```python
from build123d import *

# Parameters (mm, degrees)
AXIAL_PROFILE_MM_W     = 4
AXIAL_PROFILE_MM_H     = 19
AXIAL_HOLES_DEPTH      = 151.487507787
AXIAL_HOLES_DEPTH_BACK = 151.487507787
SKETCH2_R              = 1.25
SKETCH2_R_2            = 1.65


with BuildPart() as part:
    # Axial profile (mm) → Full revolution (revolve)
    with BuildSketch(Plane.XY, mode=Mode.PRIVATE) as full_revolution_sk:
        with Locations((133.7, 36.5)):
            Rectangle(AXIAL_PROFILE_MM_W, AXIAL_PROFILE_MM_H)
    revolve(full_revolution_sk.sketch.rotate(Axis((-110, 0, 0), (1, 0, 0)), 90), axis=Axis((-110, 0, 0), (1, 0, 0)))

    # Sketch2 → Axial holes (cut, two sides: drawn at the far end of the back side and taken through both)
    with BuildSketch(Plane(origin=(0, 0, 0), x_dir=(0, 0, -1), z_dir=(1, 0, 0)).offset(-AXIAL_HOLES_DEPTH_BACK)):
        with Locations((0, 42.2)):
            Circle(SKETCH2_R)
        with Locations((-36.54627204, -21.1)):
            Circle(SKETCH2_R)
        with Locations((36.54627204, -21.1)):
            Circle(SKETCH2_R)
        with Locations((-28.145825623, 16.25)):
            Circle(SKETCH2_R_2)
        with Locations((0, -32.5)):
            Circle(SKETCH2_R_2)
        with Locations((28.145825623, 16.25)):
            Circle(SKETCH2_R_2)
    extrude(amount=AXIAL_HOLES_DEPTH + AXIAL_HOLES_DEPTH_BACK, mode=Mode.SUBTRACT)


solid = part.part
```
Work out the finished part from the listing and answer in its coordinate system (mm). Give positions to 0.01 mm unless a question says otherwise; leave off trailing zeros. Write each loop counter-clockwise with the first axis right and the second up, starting at its lowest first coordinate (ties: lowest second). Pieces come first, ordered by that corner, then holes.
(1) The mould has two halves that part along Y. Classify faces 1 (the flat face through (131.7, 20, -20)), 2 (the cylindrical face through (133.672, -20.725, -37.739)), 3 (the cylindrical face through (133.67, 16.75, -29.72)), 4 (the cylindrical face through (133.73, -45.61, -5.99)): pulls with the +Y half, pulls with the -Y half, needs draft (parallel to the pull), parting line crosses it, or undercut.
Final values:
face 1: needs draft
face 2: undercut
face 3: undercut
face 4: parting line crosses it
(2) The part is cut by section D-D on y = 16.25. Write down the section's boundary in (x, z), plus the area to 3 significant figures.
Final values:
outline: (131.7, -43.03) - (135.7, -43.03) - (135.7, -29.8) - (131.7, -29.8) - close; (131.7, -26.5) - (135.7, -26.5) - (135.7, -21.56) - (131.7, -21.56) - close; (131.7, 21.56) - (135.7, 21.56) - (135.7, 26.5) - (131.7, 26.5) - close; (131.7, 29.8) - (135.7, 29.8) - (135.7, 43.03) - (131.7, 43.03) - close
area: 145 mm2
(3) The part is cut by section B-B on x = 133.3. Write down the section's boundary in (y, z), plus the area to 3 significant figures.
Final values:
outline: circle Ø92 at (0, 0); hole circle Ø3.3 at (-32.5, 0); hole circle Ø54 at (0, 0); hole circle Ø2.5 at (-21.1, -36.55); hole circle Ø2.5 at (-21.1, 36.55); hole circle Ø3.3 at (16.25, -28.15); hole circle Ø3.3 at (16.25, 28.15); hole circle Ø2.5 at (42.2, 0)
area: 4,320 mm2
(4) Straight lines are drawn through the part: line 1 (Y direction, x = 132.8, z = 0); line 2 (Y direction, x = 132.7, z = -1); line 3 (Z direction, x = 132.7, y = -21.1). For each, find the intervals that lie inside material, in ascending order.
Final values:
line 1: y = -46 to -34.15, -30.85 to -27, 27 to 40.95, 43.45 to 46
line 2: y = -45.99 to -33.81, -31.19 to -26.98, 26.98 to 41.45, 42.95 to 45.99
line 3: z = -40.88 to -37.8, -35.3 to -16.85, 16.85 to 35.3, 37.8 to 40.88
(5) Flat-ended cylindrical pins translate along their axes: pin 1 Ø1 at (x, y) = (134, 13) entering from +Z; pin 2 Ø1.5 at (x, y) = (135, 13.5) entering from +Z; pin 3 Ø1.5 at (x, y) = (133, -21.5) entering from +Z. Find the tip coordinate at first contact, or state that the pin passes through.
Final values:
pin 1: stops at z = 44.27
pin 2: stops at z = 44.2
pin 3: stops at z = 41.05
(6) The part is cut by section A-A on y = 0. Write down the section's boundary in (x, z), plus the area to 3 significant figures.
Final values:
outline: (131.7, -46) - (135.7, -46) - (135.7, -27) - (131.7, -27) - close; (131.7, 27) - (135.7, 27) - (135.7, 46) - (131.7, 46) - close
area: 152 mm2
(7) The part is cut by section C-C on z = -3.5. Write down the section's boundary in (x, y).
Final values:
outline: (131.7, -45.87) - (135.7, -45.87) - (135.7, -26.77) - (131.7, -26.77) - close; (131.7, 26.77) - (135.7, 26.77) - (135.7, 45.87) - (131.7, 45.87) - close
